Can you work these out from the model? Positions are in its coordinate system, mm. Face numbers are marked on the shaded views. A direction names the side the tool comes from. Round coordinates to 2 decimals unless told otherwise and drop trailing zeros. Loops run counter-clockwise (first coordinate to the right, second up) from the corner with the lowest first, then second, coordinate; pieces in that order, holes last.
(1) Which directions (+Z, -Z, +X, -X, +Y, -Y) give clear straight access to the entire face, cutting with the end or side of a thin tool? Please do the marked faces 5 and 6.
(2) Thinking about a two-plate mould opening in X: for the marked faces 1, 2, 3 and 4, which applies, released by +X, released by -X, zero draft, split by the parting line, or undercut?
(3) Will these pins go through, and if not, where does the flat tip stop? pin 1 Ø3 at (x, z) = (-7.5, 17) entering from +Y; pin 2 Ø4 at (y, z) = (21.5, 20) entering from -X; pin 3 Ø2.5 at (x, z) = (-7.5, 17) entering from -Y.
(4) If I drill on line 1 along X through (y, z) = (25.6, 8); line 2 along X through (y, z) = (25.4, 8); line 3 along X through (y, z) = (8.5, 4.25), over which ranges is the centre line in solid material (lowest first)?
(5) I want a section at C-C on z = 7.5. Write out the boundary of the cut face in (x, y).
(6) I want a section at D-D on y = 10.75. Write out the boundary of the cut face in (x, z), plus the area to 3 significant figures.
(7) I want a section at A-A on z = 17. Write out the boundary of the cut face in (x, y), plus the area to 3 significant figures.
(8) I want a section at B-B on x = -6.5. Write out the boundary of the cut face in (y, z), plus the area to 3 significant figures.
from build123d import *

# Parameters (mm, degrees)
BOSS_EXTRUDE1_DEPTH = 25
SKETCH2_R           = 2
CUT_EXTRUDE1_DEPTH  = 5


with BuildPart() as part:
    # Sketch1 → Boss-Extrude1 (new body)
    with BuildSketch(Plane.XY):
        Polygon((0, 0), (-14, 27), (0, 27), align=None)
    extrude(amount=BOSS_EXTRUDE1_DEPTH)

    # Sketch2 → Cut-Extrude1 (cut)
    with BuildSketch(Plane(origin=(0, 27, 0), x_dir=(1, 0, 0), z_dir=(0, 1, 0))):
        with Locations(Location((-7.5, -8, 0), (0, 0, 270))):
            Circle(SKETCH2_R)
        with Locations(Location((-7.5, -17, 0), (0, 0, 270))):
            Circle(SKETCH2_R)
    extrude(amount=-CUT_EXTRUDE1_DEPTH, mode=Mode.SUBTRACT)


solid = part.part
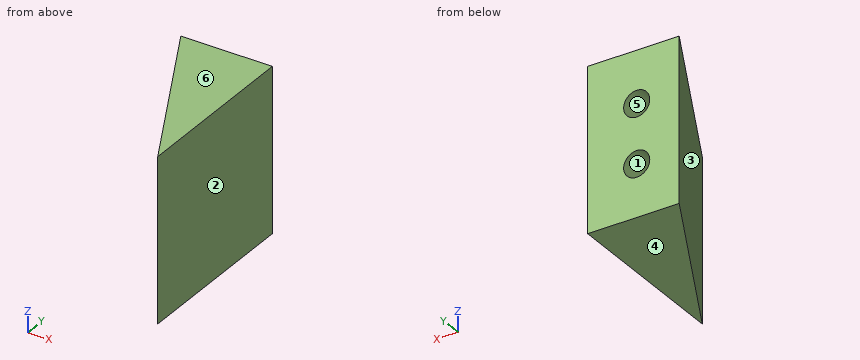
Filled sheet:
1. face 5: +Y
1. face 6: +Z, +X, -X, +Y, -Y
2. face 1: undercut
2. face 2: released by +X
2. face 3: released by -X
2. face 4: zero draft
3. pin 1: stops at y = 22
3. pin 2: stops at x = -12.19
3. pin 3: stops at y = 12.05
4. line 1: x = -13.27 to -9.5, -5.5 to 0
4. line 2: x = -13.17 to -9.5, -5.5 to 0
4. line 3: x = -4.41 to 0
5. outline: (-14, 27) - (0, 0) - (0, 27) - (-5.56, 27) - (-5.56, 22) - (-9.44, 22) - (-9.44, 27) - close
6. outline: (-5.57, 0) - (0, 0) - (0, 25) - (-5.57, 25) - close
6. area: 139 mm2
7. outline: (-14, 27) - (0, 0) - (0, 27) - (-5.5, 27) - (-5.5, 22) - (-9.5, 22) - (-9.5, 27) - close
7. area: 169 mm2
8. outline: (12.54, 0) - (27, 0) - (27, 6.27) - (22, 6.27) - (22, 9.73) - (27, 9.73) - (27, 15.27) - (22, 15.27) - (22, 18.73) - (27, 18.73) - (27, 25) - (12.54, 25) - close
8. area: 327 mm2
